Input: dimensioned drawing with shaded views. Units: mm. Origin: part minimum x, y, z. A direction names the side the tool comes from. Round coordinates to 2 decimals unless told otherwise and drop trailing zeros. Loops run counter-clockwise (first coordinate to the right, second up) from the corner with the lowest first, then second, coordinate; pieces in that order, holes last. Notation, with made-up numbers: (38, 45) - (65, 45) arc R16 ccw to (65, 58) - close; hole circle Ø1 at (57.25, -14.75). An arc over 180 degrees is marked (long way). Answer as CSV lines item,"result".
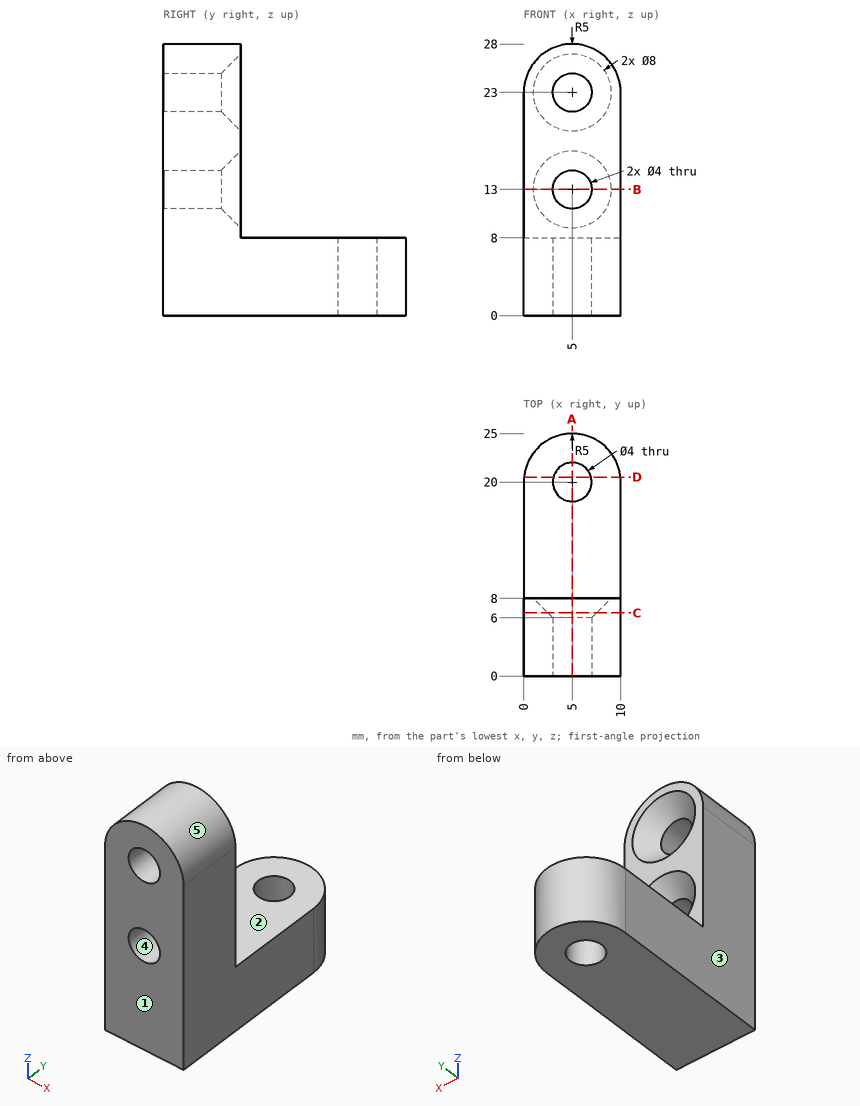
(1) Section A-A (x = 5). Output: boundary loops of the cut face in (y, z).
Findings below:
outline,"(0, 0) - (18, 0) - (18, 8) - (8, 8) - (8, 9) - (6, 11) - (0, 11) - close; (0, 15) - (6, 15) - (8, 17) - (8, 19) - (6, 21) - (0, 21) - close; (0, 25) - (6, 25) - (8, 27) - (8, 28) - (0, 28) - close; (22, 0) - (25, 0) - (25, 8) - (22, 8) - close"
(2) Material intervals for line 1 along X through (y, z) = (4.65, 23); line 2 along Z through (x, y) = (3, 6.5); line 3 along Z through (x, y) = (2.5, 7.5), sorted ascending.
Findings below:
line 1,"0 to 3, 7 to 10"
line 2,"0 to 11.5, 14.5 to 21.5, 24.5 to 27.58"
line 3,"0 to 10.55, 15.45 to 20.55, 25.45 to 27.33"
(3) Section B-B (z = 13). Output: boundary loops of the cut face in (x, y).
Findings below:
outline,"(0, 0) - (3, 0) - (3, 6) - (1, 8) - (0, 8) - close; (7, 0) - (10, 0) - (10, 8) - (9, 8) - (7, 6) - close"
(4) Access query for the marked faces 1 and 2. Directions: +Z, -Z, +X, -X, +Y, -Y. A direction counts if a zero-diameter tool reaches every point of the face in a straight line with its end or side. Return the directions, or none.
Findings below:
face 1,"+Z, -Z, +X, -X, -Y"
face 2,"+Z, +X, -X, +Y"
(5) Pin query (flat end, axial travel): P1, Ø3, axis at y = 8, z = 25, coming from the +X side; P2, Ø6, axis at x = 1, y = 19, coming from the -Z side; P3, Ø1.5, axis at x = 6, y = 11, coming from the +Z side; P4, Ø1, axis at x = 6.5, z = 15, coming from the +Y side. Return the tip coordinate at first contact, or that it passes through.
Findings below:
P1,"x = 9.97"
P2,"z = 0"
P3,"z = 8"
P4,"y = 7"
(6) Section C-C (y = 6.5). Output: boundary loops of the cut face in (x, z), and give its area (3 significant figures).
Findings below:
outline,"(0, 0) - (10, 0) - (10, 23) arc R5 ccw to (0, 23) - close; hole circle Ø5 at (5, 13); hole circle Ø5 at (5, 23)"
area,"230 mm2"
(7) Draft query along X for the marked faces 3, 4 and 5. Return one class per face: pulls with the +X half, pulls with the -X half, needs draft (parallel to the pull), parting line crosses it, or undercut.
Findings below:
face 3,"pulls with the -X half"
face 4,"undercut"
face 5,"parting line crosses it"
(8) Section D-D (y = 20.5). Output: boundary loops of the cut face in (x, z), and give its area (3 significant figures).
Findings below:
outline,"(0.03, 0) - (3.06, 0) - (3.06, 8) - (0.03, 8) - close; (6.94, 0) - (9.97, 0) - (9.97, 8) - (6.94, 8) - close"
area,"48.6 mm2"
